Verification items for the finished model (mm, model axes). A direction names the side the tool comes from. Coordinates: 2 decimals unless noted, no trailing zeros. Loops run counter-clockwise (first coordinate to the right, second up) from the corner with the lowest first, then second, coordinate; pieces in that order, holes last. Notation, with made-up numbers: (9.25, 7.25) - (31.25, 7.25) arc R28 ccw to (31.25, 42.25) - close; hole circle Ø7 at (-0.75, 78.25). An arc over 180 degrees is marked (long way). One line per item, written item: value. Start each with the question number.
(1) Gauge pin test, flat ends, axial feed: P1, Ø1.5, axis at x = -25.5, z = 2, coming from the -Y side; P2, Ø1.5, axis at y = -9.5, z = -1.5, coming from the -X side; P3, Ø0.9, axis at y = 9, z = -2, coming from the +X side. Record the tip position at first contact, or that the pin passes through.
(2) Set-up check for faces 4 (the face through (18, -7.5, -2)), 5 (the face through (15.75, -8, -1)), 6 (the face through (-18.82, 15.6, 1.48)), 7 (the face through (-21.62, 31.97, 2.04)), 8 (the face through (15.75, 8, -1)): record each of +Z, -Z, +X, -X, +Y, -Y from which the full face is reachable in a straight line by a thin tool's end or side.
(3) Section check A-A (x = 11). Record the boundary of the cut face in (y, z), plus the area to 3 significant figures.
(4) Thickness scan on probe 1 along Y at (x, z) = (4.5, 1.75); probe 2 along X at (y, z) = (-32.55, 1.5); probe 3 along Z at (x, y) = (-4.5, 19.5). Record the ranges inside material, lowest first. Write a range as [from, to].
(5) Section check B-B (y = -21.5). Record the boundary of the cut face in (x, z), plus the area to 4 significant figures.
(6) Draft check along Y on faces 1 (the face through (-5, -34, 2)), 2 (the face through (9, 15, 1)), 3 (the face through (17.75, -8, -1)). Enter one of: +Y half, -Y half, draft (parallel to the pull), parting line (faces both ways), or undercut.
```python
from build123d import *

# Parameters (mm, degrees)
SKETCH_1_W          = 36.5
SKETCH_1_H          = 68
EXTRUDE_1_DEPTH     = 3
SKETCH_2_R          = 2.5
EXTRUDE_2_DEPTH     = 4
EXTRUDE_START       = -4
EXTRUDE_3_DEPTH     = 4
CUT_EXTRUDE_START   = -4
SKETCH_4_R          = 2.5
CUT_EXTRUDE_1_DEPTH = 4
SKETCH_5_W          = 3
SKETCH_5_H          = 15
EXTRUDE_4_DEPTH     = 4
CUT_EXTRUDE_2_DEPTH = 2
SKETCH_7_R          = 2
CUT_EXTRUDE_3_DEPTH = 5
EXTRUDE_5_DEPTH     = 1
SKETCH_9_W          = 10
SKETCH_9_H          = 30
EXTRUDE_6_DEPTH     = 3
FILLET_1_R          = 2
FILLET_2_R          = 1


with BuildPart() as part:
    # 草图1 → 凸台-拉伸1 (new body)
    with BuildSketch(Plane.XY):
        Rectangle(SKETCH_1_W, SKETCH_1_H)
    extrude(amount=EXTRUDE_1_DEPTH)

    # 草图2 → 凸台-拉伸2 (add)
    with BuildSketch(Plane.XZ.offset(34)):
        with BuildLine():
            Line((-18.25, 3), (-18.25, 0))
            ThreePointArc((-18.25, 0), (-19.83113883, -0.325765386), (-21.15473751, -1.25))
            ThreePointArc((-21.15473751, -1.25), (-28.059475019, 1.5), (-21.15473751, 4.25))
            ThreePointArc((-21.15473751, 4.25), (-19.83113883, 3.325765386), (-18.25, 3))
        make_face()
        with Locations(Location((-24.059475019, 1.5, 0), (0, 0, 270))):
            Circle(SKETCH_2_R, mode=Mode.SUBTRACT)
    extrude(amount=-EXTRUDE_2_DEPTH)

    # 草图3 → 凸台-拉伸3 (add)
    with BuildSketch(Plane(origin=(0, 34, 0), x_dir=(1, 0, 0), z_dir=(0, 1, 0)).offset(EXTRUDE_START)):
        with BuildLine():
            Line((-18.25, -3), (-18.25, 0))
            ThreePointArc((-18.25, 0), (-19.83113883, 0.325765386), (-21.15473751, 1.25))
            ThreePointArc((-21.15473751, 1.25), (-28.059475019, -1.5), (-21.15473751, -4.25))
            ThreePointArc((-21.15473751, -4.25), (-19.83113883, -3.325765386), (-18.25, -3))
        make_face()
    extrude(amount=EXTRUDE_3_DEPTH)

    # 草图4 → 切除-拉伸1 (cut)
    with BuildSketch(Plane(origin=(0, 34, 0), x_dir=(1, 0, 0), z_dir=(0, 1, 0)).offset(CUT_EXTRUDE_START)):
        with Locations(Location((-24.059475019, -1.5, 0), (0, 0, 90))):
            Circle(SKETCH_4_R)
    extrude(amount=CUT_EXTRUDE_1_DEPTH, mode=Mode.SUBTRACT)

    # 草图5 → 凸台-拉伸4 (add)
    with BuildSketch(Plane(origin=(0, 0, 0), x_dir=(-1, 0, 0), z_dir=(0, 0, -1))):
        with Locations((-16.75, 0)):
            Rectangle(SKETCH_5_W, SKETCH_5_H)
    extrude(amount=EXTRUDE_4_DEPTH)

    # 草图6 → 切除-拉伸2 (cut)
    with BuildSketch(Plane(origin=(0, 0, 0), x_dir=(-1, 0, 0), z_dir=(0, 0, -1))):
        Polygon((-15.25, 7.5), (-15.25, 15), (-3.25, 15), (-3.25, -15), (-15.25, -15), (-15.25, -7.5), align=None)
    extrude(amount=-CUT_EXTRUDE_2_DEPTH, mode=Mode.SUBTRACT)

    # 草图7 → 切除-拉伸3 (cut)
    with BuildSketch(Plane(origin=(18.25, 0, 0), x_dir=(0, 0, -1), z_dir=(1, 0, 0))):
        with Locations((1, 0)):
            Circle(SKETCH_7_R)
    extrude(amount=-CUT_EXTRUDE_3_DEPTH, mode=Mode.SUBTRACT)

    # 草图8 → 凸台-拉伸5 (add, symmetric)
    with BuildSketch(Plane.ZY.offset(-16.75)):
        Polygon((-3, 7.5), (0, 10.5), (0, 7.5), align=None)
    extrude_5 = extrude(amount=EXTRUDE_5_DEPTH, both=True)

    # 镜向1: 凸台-拉伸5 across plane
    add(extrude_5.mirror(Plane.ZX))

    # 草图9 → 凸台-拉伸6 (add)
    with BuildSketch(Plane.XY.offset(3)):
        with Locations((-23.25, 0)):
            Rectangle(SKETCH_9_W, SKETCH_9_H)
    extrude(amount=-EXTRUDE_6_DEPTH)

    # 圆角1
    fillet_1_edges = [part.edges().sort_by_distance(p)[0] for p in [
        (-18.25, 15, 1.5),
        (-18.25, -15, 1.5),
    ]]
    fillet(fillet_1_edges, radius=FILLET_1_R)

    # 圆角2
    fillet_2_edges = [part.edges().sort_by_distance(p)[0] for p in [
        (15.25, 0, 2),
    ]]
    fillet(fillet_2_edges, radius=FILLET_2_R - 0.0001)  # a hair under: the kernel refuses the full size


solid = part.part
```
Responses:
1. P1: stops at y = -15
1. P2: stops at x = 15.75
1. P3: stops at x = 17.75
2. face 4: -Z, -Y
2. face 5: -Z, -X, -Y
2. face 6: +Z, -Z, -X
2. face 7: +Y
2. face 8: -Z, -X, +Y
3. outline: (-34, 0) - (-15, 0) - (-15, 2) - (15, 2) - (15, 0) - (34, 0) - (34, 3) - (-34, 3) - close
3. area: 144 mm²
4. probe 1: y = [-34, -15], [15, 34]
4. probe 2: x = [-28.06, -26.56], [-21.56, 18.25]
4. probe 3: z = [0, 3]
5. outline: (-18.25, 0) - (18.25, 0) - (18.25, 3) - (-18.25, 3) - close
5. area: 109.5 mm²
6. face 1: -Y half
6. face 2: undercut
6. face 3: draft
